Can you work these out from the model? Positions are in its coordinate system, mm. A direction names the side the tool comes from. Give positions to 0.01 mm unless a question says otherwise; leave off trailing zeros. Order: outer loops, then holes, each group sorted by start corner. A loop starts at its lowest first (then second) coordinate and runs counter-clockwise, first axis right, second up. Notation, with made-up numbers: (-4.75, 63.25) - (39.25, 63.25) arc R23 cw to (39.25, 80.25) - close; hole circle Ø2 at (56.25, 7). An arc over 180 degrees is marked (long way). Write each question's results on one line, items separated by ' | '. Start each with the question number.
Autodesk Inventor part; units mm, degrees
ref_plane "YZ Plane" through (0, 0, 0) normal (1, 0, 0) x (0, 1, 0)
ref_plane "XZ Plane" through (0, 0, 0) normal (0, 1, 0) x (-1, 0, 0)
ref_plane "XY Plane" through (0, 0, 0) normal (0, 0, 1) x (1, 0, 0)
sketch "Sketch1" plane through (0, 0, 0) normal (0, 0, 1) x (1, 0, 0)
  circle A0 centre (0, 0) radius 6.525
  line L0 (-2.0352, -3.525) -> (-4.0703, 0)
  line L1 (-4.0703, 0) -> (-2.0352, 3.525)
  line L2 (-2.0352, 3.525) -> (2.0352, 3.525)
  line L3 (2.0352, 3.525) -> (4.0703, 0)
  line L4 (4.0703, 0) -> (2.0352, -3.525)
  line L5 (2.0352, -3.525) -> (-2.0352, -3.525)
  line L6 (-4.0703, 0) -> (4.0703, 0) construction
  arc A1 (25, -2.5) -> (25, 2.5) centre (25, 0) ccw
  circle A2 centre (17.2205, -3.3329) radius 6.096
  line L7 (25, 2.5) -> (18.992, 2.5)
  line L8 (6.0271, 2.5) -> (15.449, 2.5)
  line L9 (6.0271, -2.5) -> (11.1817, -2.5)
  line L10 (23.2593, -2.5) -> (25, -2.5)
  dimension "d0" = 7.05
  dimension "d1" = 3
  dimension "d7" = 5
  dimension "d11" = 25
  dimension "d12" = 12.192
  dimension "d13" = 5.8329
  dimension "d14" = 7.7795
extrude "Extrusion2" add sketch "Sketch1" along normal blind 12
properties part number "wingnut"
Q1. If we section it at D-D (x = 20): Please give me the cut outline in (y, z).
Q2. Will these pins go through, and if not, where does the flat tip stop? P1, Ø5, axis at x = 23.5, z = 9, coming from the +Y side; P2, Ø1.5, axis at x = 8.5, z = 6.5, coming from the -Y side; P3, Ø1.5, axis at x = 6, z = 6.5, coming from the -Y side; P4, Ø5, axis at x = -0.5, y = 0, coming from the +Z side.
Q3. Which directions (+Z, -Z, +X, -X, +Y, -Y) give clear straight access to the entire face, cutting with the end or side of a thin tool? Please do faces 1 (the flat face through (11, 2.5, 6)), 2 (the flat face through (22, 2.5, 6)), 3 (the flat face through (0, -3.525, 6)).
Q4. If I drill on probe 1 along X at (y, z) = (-3, 0.5); probe 2 along X at (y, z) = (3, 2.25); probe 3 along Y at (x, z) = (10, 8.25), over which ranges is the centre line in solid material (lowest first)? Write a range as from..to.
Q5. Thinking about a two-plate mould opening in X: for faces 4 (the flat face through (10, -1, 0)), 5 (the flat face through (0, 3.525, 6)), 6 (the cylindrical face through (27.5, 0.1, 5.9)), 7 (the cylindrical face through (17.366, -9.427, 5.916)), which applies, released by +X, released by -X, zero draft, split by the parting line, or undercut?
Q6. If we section it at A-A (x = 0): Please give me the cut outline in (y, z) (3 decimals).
Q7. If we section it at B-B (y = -4): Please give me the cut outline in (x, z).
Findings below:
1) outline: (-8.76, 0) - (2.5, 0) - (2.5, 12) - (-8.76, 12) - close
2) P1: stops at y = 2.5 | P2: stops at y = -2.5 | P3: stops at y = -3.87 | P4: passes through
3) face 1: +Z, -Z, +Y | face 2: +Z, -Z, +X, +Y | face 3: +Z, -Z
4) probe 1: x = -5.79..-2.34, 2.34..5.79, 11.13..23.31 | probe 2: x = -5.79..-2.34, 2.34..5.79 | probe 3: y = -2.5..2.5
5) face 4: zero draft | face 5: undercut | face 6: released by +X | face 7: undercut
6) outline: (-6.525, 0) - (-3.525, 0) - (-3.525, 12) - (-6.525, 12) - close; (3.525, 0) - (6.525, 0) - (6.525, 12) - (3.525, 12) - close
7) outline: (-5.16, 0) - (5.16, 0) - (5.16, 12) - (-5.16, 12) - close; (11.16, 0) - (23.28, 0) - (23.28, 12) - (11.16, 12) - close
